Autodesk Inventor part; units mm, degrees
ref_plane "Plan YZ" through (0, 0, 0) normal (1, 0, 0) x (0, 1, 0)
ref_plane "Plan XZ" through (0, 0, 0) normal (0, 1, 0) x (-1, 0, 0)
ref_plane "Plan XY" through (0, 0, 0) normal (0, 0, 1) x (1, 0, 0)
sketch "Esquisse1" plane through (0, 0, 0) normal (0, 0, 1) x (1, 0, 0)
  circle A0 centre (0, 0) radius 1.425
  dimension "d0" = 2.85
extrude "Extrusion1" add sketch "Esquisse1" along normal blind 3
sketch "Esquisse6" plane through (0, 0, 3) normal (0, 0, 1) x (1, 0, 0)
  line L0 (-4.8497, 0) -> (4.8497, 0) construction
  line L1 (0, -4.2) -> (0, 4.2) construction
  line L2 (-1.7321, -3) -> (-3.4641, 0)
  line L3 (-3.4641, 0) -> (-1.7321, 3)
  line L4 (-1.7321, 3) -> (0, 3)
  line L5 (-1.7321, -3) -> (0, -3)
  line L6 (1.7321, -3) -> (3.4641, 0)
  line L7 (3.4641, 0) -> (1.7321, 3)
  line L8 (1.7321, 3) -> (0, 3)
  line L9 (1.7321, -3) -> (0, -3)
  point P0 (0, 0)
  dimension "d4" = 6
  dimension "d8" = 120
  dimension "d10" = 6
extrude "Extrusion2" add sketch "Esquisse6" along normal blind 25
sketch "Esquisse7" plane through (0, 0, 28) normal (0, 0, 1) x (1, 0, 0)
  circle A0 centre (0, 0) radius 1.425
hole "Perçage1" at (0, 0, 28) direction (0, 0, -1) diameter 2.459 depth 8.5 tip angle 118
thread "Filetage1"
properties part number "entretoise25" material "."
Input: part model. Units: mm. Frame: model coordinates. A direction names the side the tool comes from. Round coordinates to 2 decimals unless told otherwise and drop trailing zeros. Loops run counter-clockwise (first coordinate to the right, second up) from the corner with the lowest first, then second, coordinate; pieces in that order, holes last. Notation, with made-up numbers: (49, 28.25) -> (88, 28.25) arc R26 ccw to (88, 42.25) -> close; hole circle Ø9 at (-18, 26.25). An arc over 180 degrees is marked (long way). Answer as a JSON object with one key per item and string values. Group by question number.
1) Section query B-B on z = 15. Output: boundary loops of the cut face in (x, y), plus the area to 3 significant figures.
2) Draft query along Y for faces 3 (the flat face through (1.5, 0.7, 3)), 4 (the cylindrical face through (0.748, 0.976, 23.69)), 5 (the conical face through (-0.21, 0.05, 18.89)), 6 (the flat face through (-2.6, 1.5, 15.3)). Return one class per face: +Y half, -Y half, draft (parallel to the pull), parting line (faces both ways), or undercut.
3) Section query D-D on x = 3. Output: boundary loops of the cut face in (y, z).
4) Ray query, L1, parallel to Y at x = 0, z = 25.5; L2, parallel to Z at x = 2.5, y = 1.3; L3, parallel to Y at x = 0.75, z = 25. Return the intervals inside material, ascending.
5) Reachability of faces 1 (the flat face through (2.6, -1.5, 15.3)), 2 (the cylindrical face through (-1.13, 0.87, 1.48)) from +Z, -Z, +X, -X, +Y, -Y: full face, straight path, thin tool, end or side. Return the list, or none.
6) Section query C-C on y = -2.35. Output: boundary loops of the cut face in (x, z), plus the area to 3 significant figures.
7) Section query A-A on z = 26. Output: boundary loops of the cut face in (x, y), plus the area to 3 significant figures.
Reply:
{
 "1": {"outline": "(-3.46, 0) -> (-1.73, -3) -> (1.73, -3) -> (3.46, 0) -> (1.73, 3) -> (-1.73, 3) -> close", "area": "31.2 mm2"},
 "2": {"face 3": "draft", "face 4": "undercut", "face 5": "undercut", "face 6": "+Y half"},
 "3": {"outline": "(-0.8, 3) -> (0.8, 3) -> (0.8, 28) -> (-0.8, 28) -> close"},
 "4": {"L1": "y = -3 to -1.23, 1.23 to 3", "L2": "z = 3 to 28", "L3": "y = -3 to -0.97, 0.97 to 3"},
 "5": {"face 1": "+Z, -Z, +X, -Y", "face 2": "-Z"},
 "6": {"outline": "(-2.11, 3) -> (2.11, 3) -> (2.11, 28) -> (-2.11, 28) -> close", "area": "105 mm2"},
 "7": {"outline": "(-3.46, 0) -> (-1.73, -3) -> (1.73, -3) -> (3.46, 0) -> (1.73, 3) -> (-1.73, 3) -> close; hole circle Ø2.46 at (0, 0)", "area": "26.4 mm2"}
}
